Verification items for this drawing (mm, ordinates from the low corner). Coordinates: 2 decimals unless noted, no trailing zeros. Write each loop counter-clockwise with the first axis right and the second up, starting at its lowest first coordinate (ties: lowest second). Pieces come first, ordered by that corner, then holes. Notation, with made-up numbers: (77.5, -10.75) -> (84.5, -10.75) arc R23 ccw to (84.5, 0.25) -> close; hole circle Ø11 at (31.5, 28.25). An arc over 180 degrees is marked (long way). Use CSV: the item, a comma, the result in double quotes.
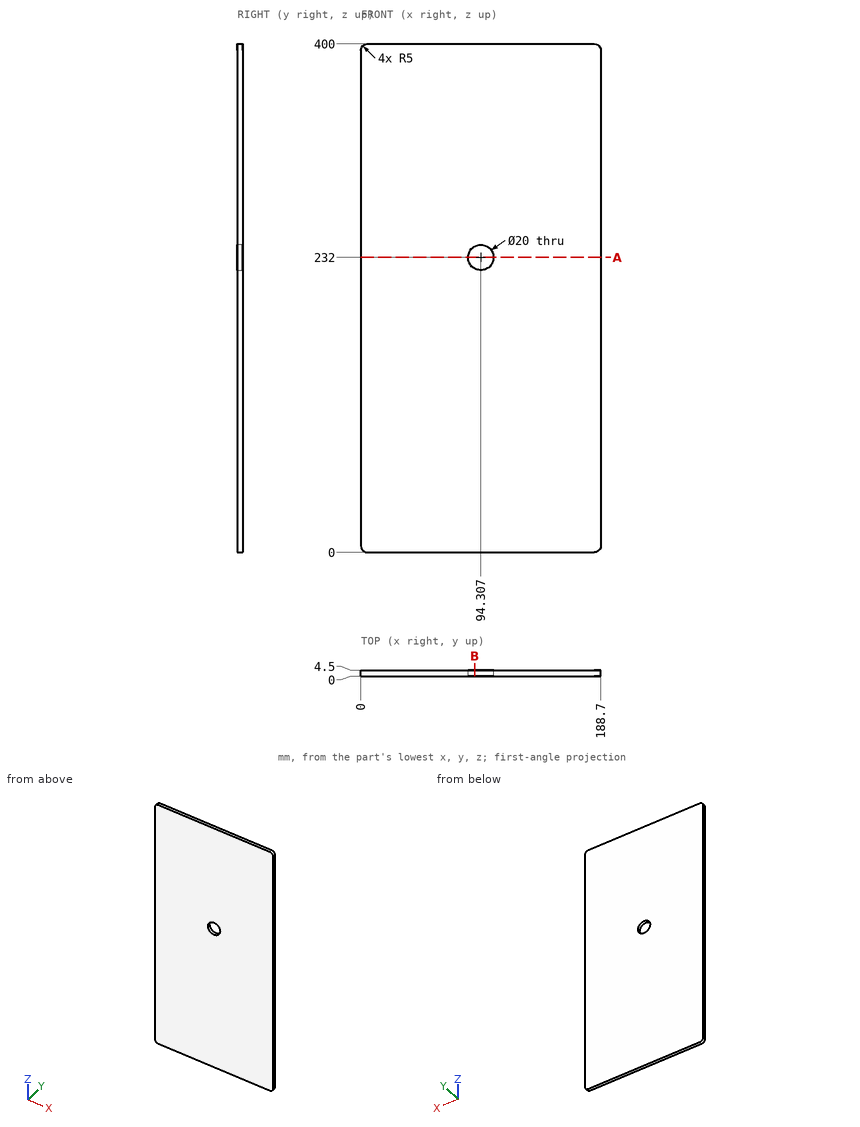
1) Cross-section at A-A (z = 232). Record the boundary of the cut face in (x, y), plus the area to 3 significant figures.
Return value:
outline,"(0, 0) -> (84.31, 0) -> (84.31, 4.5) -> (0, 4.5) -> close; (104.31, 0) -> (188.7, 0) -> (188.7, 4.5) -> (104.31, 4.5) -> close"
area,"759 mm2"
2) Cross-section at B-B (x = 89.5). Record the boundary of the cut face in (y, z), plus the area to 3 significant figures.
Return value:
outline,"(0, 0) -> (4.5, 0) -> (4.5, 223.23) -> (0, 223.23) -> close; (0, 240.77) -> (4.5, 240.77) -> (4.5, 400) -> (0, 400) -> close"
area,"1,720 mm2"
3) Scan lines: L1, parallel to X at y = 1.05, z = 232; L2, parallel to Z at x = 87, y = 2.9 (1 decimal). Record each from-to range of solid material in increasing order.
Return value:
L1,"0 to 84.31, 104.31 to 188.7"
L2,"0 to 225.2, 238.8 to 400"
